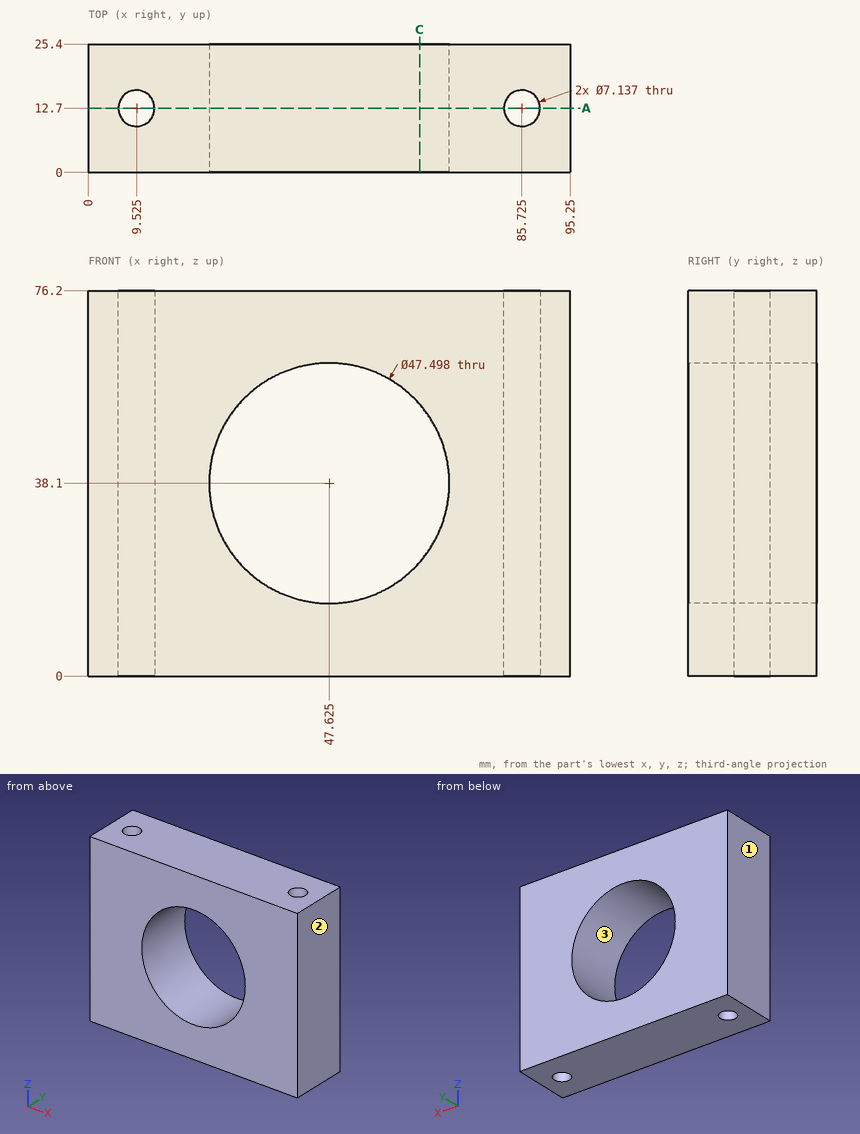
Study the drawing (mm; zero at the part's minimum x, y, z) and answer. Coordinates: 2 decimals unless noted, no trailing zeros. Loops run counter-clockwise (first coordinate to the right, second up) from the corner with the lowest first, then second, coordinate; pieces in that order, holes last. Notation, with made-up numbers: M 73.25,-6 L 78.25,-6 A13 ccw 78.25,2 Z; hole C -37.5,25.25 d10. An arc over 180 degrees is marked long. Answer in a Markdown table with one row per item. Add a question column.
1. The mould has two halves that part along X. Classify the marked faces 1, 2 and 3: pulls with the +X half, pulls with the -X half, needs draft (parallel to the pull), parting line crosses it, or undercut.
2. Consider L1, parallel to Z at x = 48.5, y = 23.75; L2, parallel to Y at x = 8, z = 10 (1 decimal); L3, parallel to Y at x = 84, z = 11.5 (1 decimal). Determine where each line is inside the solid, lowest interval first.
3. Find section C-C, the plane x = 65.5. Write down the section's boundary in (y, z).
4. Find section A-A, the plane y = 12.7. State how many separate pieces and enclosed holes the cut face has, then the cut area to 3 significant figures.
Reported:
| question | item | result |
|---|---|---|
| 1 | face 1 | pulls with the -X half |
| 1 | face 2 | pulls with the +X half |
| 1 | face 3 | undercut |
| 2 | L1 | z = 0 to 14.37, 61.83 to 76.2 |
| 2 | L2 | y = 0 to 9.5, 15.9 to 25.4 |
| 2 | L3 | y = 0 to 9.6, 15.8 to 25.4 |
| 3 | outline | M 0,0 L 25.4,0 L 25.4,22.46 L 0,22.46 Z; M 0,53.74 L 25.4,53.74 L 25.4,76.2 L 0,76.2 Z |
| 4 | separate pieces | 3 |
| 4 | enclosed holes | 1 |
| 4 | area | 4,400 mm^2 |
